Source: CAD feature listing. Evaluate the final solid. Frame: model axes, mm. Face numbers are marked on the shaded views. A direction names the side the tool comes from. Coordinates: 2 decimals unless noted, no trailing zeros. Order: outer loops, then holes, each group sorted by start corner. A loop starts at its lowest first (then second) coordinate and runs counter-clockwise, first axis right, second up.
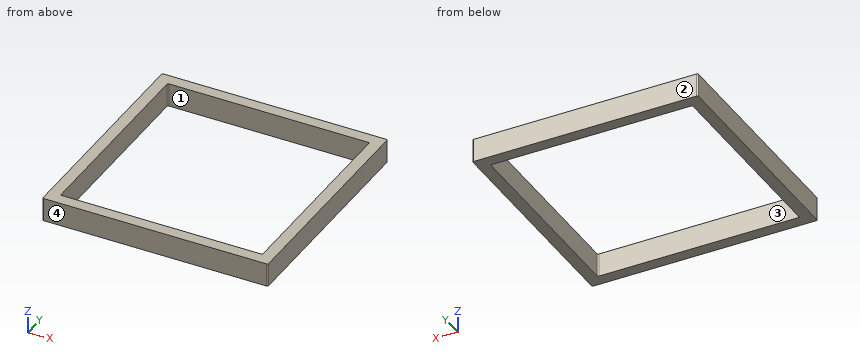
Autodesk Inventor part; units mm, degrees
ref_plane "YZ Plane" through (0, 0, 0) normal (1, 0, 0) x (0, 1, 0)
ref_plane "XZ Plane" through (0, 0, 0) normal (0, 1, 0) x (-1, 0, 0)
ref_plane "XY Plane" through (0, 0, 0) normal (0, 0, 1) x (1, 0, 0)
sketch "Sketch1" plane through (0, 0, 0) normal (0, 0, 1) x (1, 0, 0)
  line L0 (-36.576, 56.9271) -> (-36.576, 8.1591)
  line L1 (-36.576, 8.1591) -> (12.192, 8.1591)
  line L2 (12.192, 8.1591) -> (12.192, 56.9271)
  line L3 (12.192, 56.9271) -> (-36.576, 56.9271)
  line L4 (9.652, 10.6991) -> (-34.036, 10.6991)
  line L5 (-34.036, 10.6991) -> (-34.036, 54.3871)
  line L6 (-34.036, 54.3871) -> (9.652, 54.3871)
  line L7 (9.652, 54.3871) -> (9.652, 10.6991)
  point P0 (0, 0)
  dimension "d0" = 2.54
extrude "Extrusion1" add sketch "Sketch1" along normal blind 5.08
fillet "Fillet1" radius 0.254 8 edges at (12.192, 8.1591, 2.54) (-36.576, 8.1591, 2.54) (-36.576, 56.9271, 2.54) (12.192, 56.9271, 2.54) (-34.036, 10.6991, 2.54) (9.652, 10.6991, 2.54) (-34.036, 54.3871, 2.54) (9.652, 54.3871, 2.54)
properties part number "infTrim" material "ABS Plastic"
1. Section query B-B on y = 15.5. Return loops of the section in (x, z), plus the area to 3 significant figures.
Findings:
outline: (-36.58, 0) - (-34.04, 0) - (-34.04, 5.08) - (-36.58, 5.08) - close; (9.65, 0) - (12.19, 0) - (12.19, 5.08) - (9.65, 5.08) - close
area: 25.8 mm2
2. Draft query along X for the marked faces 3 and 4. Return one class per face: released by +X, released by -X, zero draft, split by the parting line, or undercut.
Findings:
face 3: undercut
face 4: zero draft
3. Section query A-A on z = 4. Return loops of the section in (x, y), plus the area to 3 significant figures.
Findings:
outline: (-36.58, 8.41) arc R0.25 ccw to (-36.32, 8.16) - (11.94, 8.16) arc R0.25 ccw to (12.19, 8.41) - (12.19, 56.67) arc R0.25 ccw to (11.94, 56.93) - (-36.32, 56.93) arc R0.25 ccw to (-36.58, 56.67) - close; hole (-34.04, 10.95) arc R0.25 ccw to (-33.78, 10.7) - (9.4, 10.7) arc R0.25 ccw to (9.65, 10.95) - (9.65, 54.13) arc R0.25 ccw to (9.4, 54.39) - (-33.78, 54.39) arc R0.25 ccw to (-34.04, 54.13) - close
area: 470 mm2
4. Ray query, line 1 (Y direction, x = -1, z = 0.25); line 2 (X direction, y = 51, z = 0.85). Return the intervals inside material, ascending.
Findings:
line 1: y = 8.16 to 10.7, 54.39 to 56.93
line 2: x = -36.58 to -34.04, 9.65 to 12.19
5. Access query for the marked faces 1 and 2. Directions: +Z, -Z, +X, -X, +Y, -Y. A direction counts if a zero-diameter tool reaches every point of the face in a straight line with its end or side. Return the directions, or none.
Findings:
face 1: +Z, -Z
face 2: +Z, -Z, +X, -X, +Y
6. Section query C-C on x = 1. Return loops of the section in (y, z).
Findings:
outline: (8.16, 0) - (10.7, 0) - (10.7, 5.08) - (8.16, 5.08) - close; (54.39, 0) - (56.93, 0) - (56.93, 5.08) - (54.39, 5.08) - close
